```python
from build123d import *

# Parameters (mm, degrees)
F0_W          = 28.575
F0_H          = 107.95
F1_DEPTH      = 6.35
F2_R          = 3.81
F8_DEPTH      = 15.875
F8_DEPTH_BACK = 15.875
F9_W          = 9.525
F9_H          = 6.35
F9_W_2        = 29.21
F9_H_2        = 11.43
F10_DEPTH     = 92.076
F12_DEPTH     = 7.62


with BuildPart() as f1:
    # F0 (on Top) → F1 (new body)
    with BuildSketch(Plane.XY):
        with Locations((14.2875, 53.975)):
            Rectangle(F0_W, F0_H)
    extrude(amount=F1_DEPTH)

    # F2
    f2_edges = [f1.edges().sort_by_distance(p)[0] for p in [
        (28.575, 0, 3.175),
        (0, 0, 3.175),
        (28.575, 107.95, 3.175),
        (0, 107.95, 3.175),
        (0, 53.975, 6.35),
        (14.2875, 0, 6.35),
        (28.575, 53.975, 6.35),
        (14.2875, 107.95, 6.35),
    ]]
    fillet(f2_edges, radius=F2_R)

    # F7 (on 3pt) → F8 (join, two sides)
    with BuildSketch(Plane.YZ.offset(14.2875)) as f8_sk:
        Polygon((28.575, 25.4), (15.875, 25.4), (15.875, 12.7), (47.625, 12.7), (47.625, 6.35), (53.975, 6.35), (60.325, 6.35), (60.325, 12.7), (92.075, 12.7), (92.075, 25.4), (79.375, 25.4), (79.375, 19.05), (85.725, 19.05), (85.725, 15.875), (79.375, 15.875), (79.375, 13.97), (59.055, 13.97), (59.055, 7.62), (48.895, 7.62), (48.895, 13.97), (28.575, 13.97), (28.575, 15.875), (22.225, 15.875), (22.225, 19.05), (28.575, 19.05), align=None)
    extrude(amount=-F8_DEPTH)
    extrude(f8_sk.sketch, amount=F8_DEPTH_BACK)

    # F9 (on face) → F10 (cut, through all)
    with BuildSketch(Plane.XZ.offset(-15.875)):
        with Locations((3.175, 9.525)):
            Rectangle(F9_W, F9_H)
        with Locations((14.2875, 19.685)):
            Rectangle(F9_W_2, F9_H_2)
        with Locations((25.4, 9.525)):
            Rectangle(F9_W, F9_H)
    extrude(amount=-F10_DEPTH, mode=Mode.SUBTRACT)

    # F11 (on face) → F12 (cut, through all)
    with BuildSketch(Plane.XY.offset(13.97)):
        Polygon((7.9375, 48.895), (-1.5875, 48.895), (-1.5875, 28.575), (-0.3175, 28.575), (7.9375, 28.575), align=None)
        Polygon((-0.3175, 79.375), (-1.5875, 79.375), (-1.5875, 59.055), (7.9375, 59.055), (7.9375, 79.375), align=None)
        Polygon((30.1625, 48.895), (20.6375, 48.895), (20.6375, 28.575), (28.8925, 28.575), (30.1625, 28.575), align=None)
        Polygon((20.6375, 79.375), (20.6375, 59.055), (30.1625, 59.055), (30.1625, 79.375), (28.8925, 79.375), align=None)
    extrude(amount=-F12_DEPTH, mode=Mode.SUBTRACT)


solid = f1.part
```
Geometry: final body of the model. Coordinates: model frame, mm. A direction names the side the tool comes from. Round coordinates to 2 decimals unless told otherwise and drop trailing zeros. Loops run counter-clockwise (first coordinate to the right, second up) from the corner with the lowest first, then second, coordinate; pieces in that order, holes last. Notation, with made-up numbers: (66.5, 81.25) -> (75.5, 81.25) arc R25 ccw to (75.5, 99.25) -> close; hole circle Ø11 at (-4, 0.5). An arc over 180 degrees is marked (long way). Use one line per item in the form item = value. Start each with the question number.
1) Draft query along Z for faces 4 (the cylindrical face through (27.49, 54.68, 5.2)), 5 (the flat face through (20.638, 54, 7)), 6 (the flat face through (14, 54, 7.62)). Return one class per face: released by +Z, released by -Z, zero draft, split by the parting line, or undercut.
2) Line query: L1, parallel to Z at x = 8, y = 61; L2, parallel to Y at x = 10.5, z = 12.75 (3 decimals); L3, parallel to Y at x = 15.5, z = 9.5 (3 decimals). Output: solid intervals per line, ascending.
3) Section C-C on z = 17.25. Output: boundary loops of the cut face in (x, y) (1 decimal), then the cut area to 3 significant figures.
4) First-contact query: P1, Ø1, axis at x = -1, y = 84, coming from the -Z side; P2, Ø5, axis at x = 7.5, z = 11.5, coming from the +Y side (3 decimals); P3, Ø0.6, axis at x = 29.5, z = 20.5, coming from the -Y side (3 decimals); P4, Ø5, axis at x = 18.5, y = 37, coming from the -Z side. Flat tips, straight axial feed; report the tip coordinate or a pass-through.
5) Access query for faces 1 (the flat face through (14, 48.895, 11)), 2 (the flat face through (3.1, 28.575, 13.6)), 3 (the flat face through (28.892, 22, 20)). Directions: +Z, -Z, +X, -X, +Y, -Y. A direction counts if a zero-diameter tool reaches every point of the face in a straight line with its end or side. Return the directions, or none.
6) Section B-B on y = 24.5. Give the number of separate pieces and of enclosed holes in the cut face, then the cut area to 3 significant figures.
7) Section D-D on z = 10.75. Output: boundary loops of the cut face in (x, y) (1 decimal).
Response:
q1.face_4 = undercut
q1.face_5 = zero draft
q1.face_6 = released by +Z
q2.L1 = 0 to 6.35, 12.7 to 13.97
q2.L2 = 15.875 to 48.895, 59.055 to 92.075
q2.L3 = 47.625 to 48.895, 59.055 to 60.325
q3.outline = (-1.6, 15.9) -> (-0.3, 15.9) -> (-0.3, 22.2) -> (-1.6, 22.2) -> close; (-1.6, 85.7) -> (-0.3, 85.7) -> (-0.3, 92.1) -> (-1.6, 92.1) -> close; (28.9, 15.9) -> (30.2, 15.9) -> (30.2, 22.2) -> (28.9, 22.2) -> close; (28.9, 85.7) -> (30.2, 85.7) -> (30.2, 92.1) -> (28.9, 92.1) -> close
q3.area = 32.3 mm^2
q4.P1 = 12.7
q4.P2 = 92.075
q4.P3 = 15.875
q4.P4 = 0
q5.face_1 = +Z, +X, -X
q5.face_2 = +Z, -X
q5.face_3 = +Z, +Y, -Y
q6.separate_pieces = 4
q6.enclosed_holes = 0
q6.area = 237 mm^2
q7.outline = (7.9, 47.6) -> (20.6, 47.6) -> (20.6, 48.9) -> (7.9, 48.9) -> close; (7.9, 59.1) -> (20.6, 59.1) -> (20.6, 60.3) -> (7.9, 60.3) -> close
